Could you check a few things on this model? Use its own coordinates, in mm. A direction names the side the tool comes from. Round coordinates to 2 decimals unless told otherwise and drop trailing zeros. Loops run counter-clockwise (first coordinate to the right, second up) from the corner with the lowest first, then second, coordinate; pieces in that order, holes last. Notation, with made-up numbers: (-30.75, -26.75) - (-12.75, -26.75) arc R10 ccw to (-12.75, -9.75) - close; hole circle Ø4 at (5, 58). An arc over 180 degrees is marked (long way). Answer as CSV lines item,"result". Start each with the question number.
1) Suppose I cut it at C-C, the plane y = -5. Write out the boundary of the cut face in (x, z), then the cut area to 3 significant figures.
2) Suppose I cut it at B-B, the plane x = -14. Write out the boundary of the cut face in (y, z).
3) Suppose I cut it at D-D, the plane x = 8. Count the separate pieces of the cut face and the enclosed holes in it, then the cut area to 3 significant figures.
4) Please list where these lines run through material, in increasing order: line 1 along Z through (x, y) = (9, 23.75); line 2 along X through (y, z) = (15.5, 22.5); line 3 along Z through (x, y) = (14.5, -15).
5) We'd pull the mould along Z, two halves only. Please class faces 1 (the face through (17, 12.4, 7.1)), 2 (the face through (8.685, 11.514, -22.789)), 3 (the face through (0, 1, -30)): pulls with the +Z half, pulls with the -Z half, needs draft (parallel to the pull), parting line crosses it, or undercut.
6) Which directions (+Z, -Z, +X, -X, +Y, -Y) give clear straight access to the entire face, cutting with the end or side of a thin tool? Please do faces 4 (the face through (-0.238, -5.362, 12.932)), 5 (the face through (10.95, 19.48, -21)), 6 (the face through (10.491, 12.493, -11.164)).
7) I'm going to push flat-ended pins straight in: pin 1 Ø4.5 at (x, z) = (-9, 22.5) entering from +Y; pin 2 Ø5.5 at (x, z) = (9, -22.5) entering from +Y; pin 3 Ø3 at (y, z) = (13.44, 13.44) entering from +X. Where does each tip first touch, or does it pass through?
8) Suppose I cut it at A-A, the plane z = 0. Write out the boundary of the cut face in (x, y).
```python
from build123d import *

# Parameters (mm, degrees)
SCHIZZO1_W                   = 60
SCHIZZO1_H                   = 54
ESTRUSIONE_ESTRUSIONE1_DEPTH = 34
FORO_PER_VITE_M24_1_D        = 28
FORO1_D                      = 4.917
FORO1_DEPTH                  = 14.312635171
FORO1_TIP                    = 1.419415637
FORO2_D                      = 4.917
FORO2_DEPTH                  = 12.312635171
FORO2_TIP                    = 1.419415637
SMUSSO1_SIZE                 = 0.5415
SMUSSO2_SIZE                 = 2


with BuildPart() as part:
    # Schizzo1 → Estrusione-Estrusione1 (new body)
    with BuildSketch(Plane(origin=(17, 0, 0), x_dir=(0, 0, -1), z_dir=(1, 0, 0))):
        Rectangle(SCHIZZO1_W, SCHIZZO1_H)
    extrude(amount=-ESTRUSIONE_ESTRUSIONE1_DEPTH)

    # Foro per Vite M24-1 (through all)
    with Locations(Plane(origin=(17, 0, 0), x_dir=(0, 0, -1), z_dir=(1, 0, 0))):
        with Locations((0, 0)):
            Hole(FORO_PER_VITE_M24_1_D / 2)

    # Foro1
    with Locations(Plane(origin=(0, 27, 0), x_dir=(1, 0, 0), z_dir=(0, 1, 0))):
        with Locations((9, 22.5), (9, -22.5), (-9, 22.5), (-9, -22.5)):
            Hole(FORO1_D / 2, depth=FORO1_DEPTH)
            with Locations((0, 0, -(FORO1_DEPTH + FORO1_TIP / 2))):  # 120° drill point
                Cone(0, FORO1_D / 2, FORO1_TIP, mode=Mode.SUBTRACT)

    # Foro2
    with Locations(Plane(origin=(17, 0, 0), x_dir=(0, 0, -1), z_dir=(1, 0, 0))):
        with Locations((13.435028843, 13.435028843), (-13.435028843, -13.435028843), (13.435028843, -13.435028843), (-13.435028843, 13.435028843)):
            Hole(FORO2_D / 2, depth=FORO2_DEPTH)
            with Locations((0, 0, -(FORO2_DEPTH + FORO2_TIP / 2))):  # 120° drill point
                Cone(0, FORO2_D / 2, FORO2_TIP, mode=Mode.SUBTRACT)

    # Smusso1
    smusso1_edges = [part.edges().sort_by_distance(p)[0] for p in [
        (-6.5415, 27, 22.5),
        (-6.5415, 27, -22.5),
        (11.4585, 27, 22.5),
        (11.4585, 27, -22.5),
        (17, 13.435028843, 10.976528843),
        (17, -13.435028843, -15.893528843),
        (17, -13.435028843, 10.976528843),
        (17, 13.435028843, -15.893528843),
    ]]
    chamfer(smusso1_edges, length=SMUSSO1_SIZE)

    # Smusso2
    smusso2_edges = [part.edges().sort_by_distance(p)[0] for p in [
        (0, -27, 30),
        (0, -27, -30),
    ]]
    chamfer(smusso2_edges, length=SMUSSO2_SIZE)


solid = part.part
```
Filled sheet:
1,outline,"(-17, -30) - (17, -30) - (17, -13.08) - (-17, -13.08) - close; (-17, 13.08) - (17, 13.08) - (17, 30) - (-17, 30) - close"
1,area,"1,150 mm²"
2,outline,"(-27, -28) - (-25, -30) - (27, -30) - (27, 30) - (-25, 30) - (-27, 28) - close; hole circle Ø28 at (0, 0)"
3,separate pieces,"1"
3,enclosed holes,"5"
3,area,"2,410 mm²"
4,line 1,"-30 to -24.96, -20.04 to 20.04, 24.96 to 30"
4,line 2,"-17 to -11.46, -6.54 to 6.54, 11.46 to 17"
4,line 3,"-30 to -15.33, -11.54 to 11.54, 15.33 to 30"
5,face 1,"needs draft"
5,face 2,"undercut"
5,face 3,"pulls with the -Z half"
6,face 4,"+X, -X"
6,face 5,"+Y"
6,face 6,"+X"
7,pin 1,"y = 12.57"
7,pin 2,"y = 26.75"
7,pin 3,"x = 4.14"
8,outline,"(-17, -27) - (17, -27) - (17, -14) - (-17, -14) - close; (-17, 14) - (17, 14) - (17, 27) - (-17, 27) - close"
